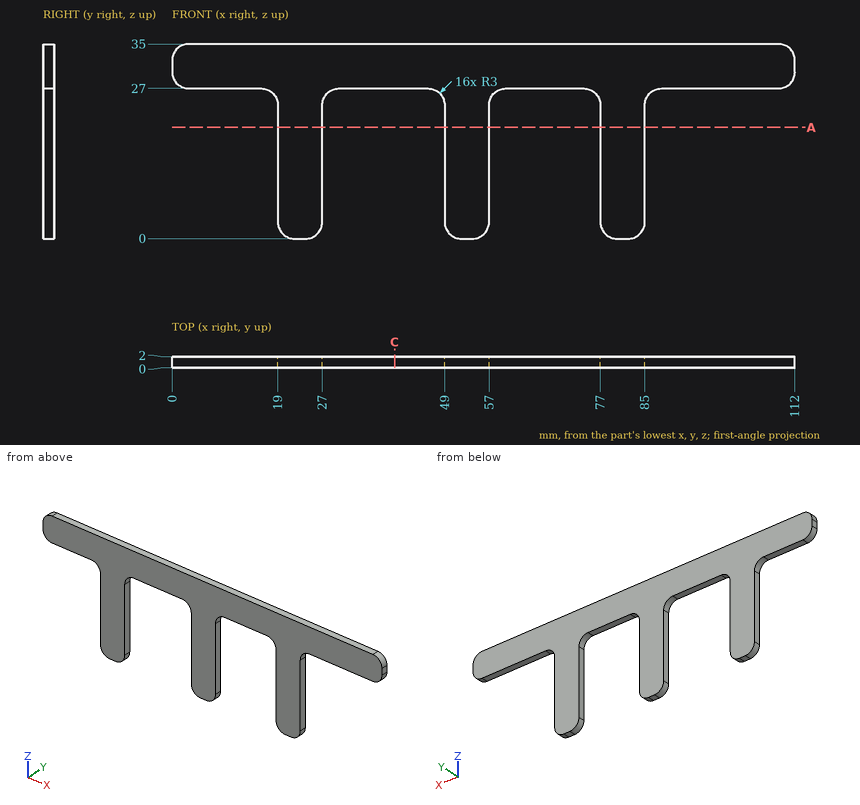
The drawing under review shows one solid part. Ordinate dimensions are in mm from its lowest x, y, z. Round coordinates to 2 decimals unless told otherwise and drop trailing zeros. Write each loop counter-clockwise with the first axis right and the second up, starting at its lowest first coordinate (ties: lowest second). Pieces come first, ordered by that corner, then holes. Notation, with made-up numbers: (-1, -27.5) - (43, -27.5) arc R21 ccw to (43, -4.5) - close; hole circle Ø2 at (70.25, -6). An arc over 180 degrees is marked (long way). Put each result on its own line as item: value.
Q1. Insertion check: pin 1 Ø12 at (x, z) = (12, 11) entering from -Y; pin 2 Ø1 at (x, y) = (65, 0.5) entering from -Z; pin 3 Ø1 at (y, z) = (1.5, 18.5) entering from +X; pin 4 Ø1 at (y, z) = (1, 15) entering from -X. Each pin has a flat end and moves straight along its axis. Give the tip position at first contact, or say it passes through.
Solved:
pin 1: passes through
pin 2: stops at z = 27
pin 3: stops at x = 85
pin 4: stops at x = 19
Q2. We need section C-C (x = 40). Give the boundary of the cut face in (y, z), and give its area (3 significant figures).
Solved:
outline: (0, 27) - (2, 27) - (2, 35) - (0, 35) - close
area: 16.0 mm2
Q3. Wall thickness on probe 1 along X at (y, z) = (1.8, 7); probe 2 along Z at (x, y) = (100, 1.1); probe 3 along X at (y, z) = (0.4, 26): over which ranges is each line inside the solid? List them lowest first.
Solved:
probe 1: x = 19 to 27, 49 to 57, 77 to 85
probe 2: z = 27 to 35
probe 3: x = 18.24 to 27.76, 48.24 to 57.76, 76.24 to 85.76
Q4. We need section A-A (z = 20). Give the boundary of the cut face in (x, y).
Solved:
outline: (19, 0) - (27, 0) - (27, 2) - (19, 2) - close; (49, 0) - (57, 0) - (57, 2) - (49, 2) - close; (77, 0) - (85, 0) - (85, 2) - (77, 2) - close
